Drawing for the job (mm, zero at the part's lowest x, y, z). Round coordinates to 2 decimals unless told otherwise and drop trailing zeros. Write each loop counter-clockwise with the first axis right and the second up, starting at its lowest first coordinate (ties: lowest second). Pieces come first, ordered by that corner, then holes.
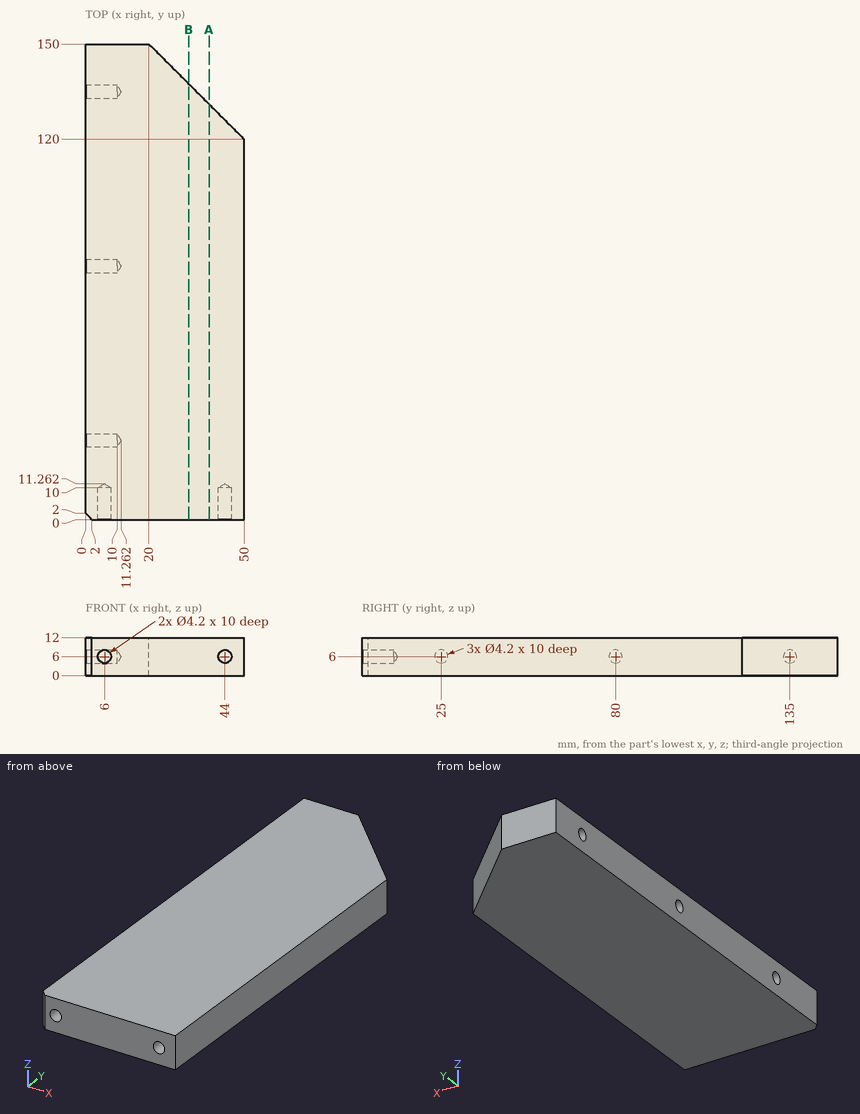
Q1. Saw through at A-A, the plane x = 39. Write the cut outline in (y, z), and give its area (3 significant figures).
Q2. Wall check: line 1 (Z direction, x = 6, y = 3); line 2 (Y direction, x = 7.25, z = 6); line 3 (Y direction, x = 48, z = 10.75). Give the ranges that are in metal, low to high.
Q3. Drop flat-ended pins along their axis: P1, Ø3.5, axis at x = 44, z = 6, coming from the -Y side; P2, Ø1.5, axis at x = 42, z = 2.5, coming from the +Y side; P3, Ø4, axis at y = 135, z = 6, coming from the -X side. Give the stop position or say it passes through.
Q4. Saw through at B-B, the plane x = 32.5. Write the cut outline in (y, z), and give its area (3 significant figures).
Computed:
1. outline: (0, 0) - (131, 0) - (131, 12) - (0, 12) - close
1. area: 1,570 mm2
2. line 1: z = 0 to 3.9, 8.1 to 12
2. line 2: y = 10.51 to 22.9, 27.1 to 77.9, 82.1 to 132.9, 137.1 to 150
2. line 3: y = 0 to 122
3. P1: stops at y = 10.21
3. P2: stops at y = 128.75
3. P3: stops at x = 10.06
4. outline: (0, 0) - (137.5, 0) - (137.5, 12) - (0, 12) - close
4. area: 1,650 mm2
